from build123d import *
from OCP.BRepFilletAPI import BRepFilletAPI_MakeChamfer

# Parameters (mm, degrees)
SKETCH1_W               = 41
SKETCH1_H               = 34.5
SKETCH1_W_2             = 35
SKETCH1_H_2             = 28.5
BOSS_EXTRUDE1_DEPTH     = 5
SKETCH2_W               = 35
SKETCH2_H               = 28.5
BOSS_EXTRUDE2_DEPTH     = 1
SKETCH6_W               = 34.5
SKETCH6_H               = 5
CUT_EXTRUDE2_DEPTH      = 3
SKETCH7_W               = 1.6
SKETCH7_H               = 3
SKETCH7_H_2             = 3.078736203
BOSS_EXTRUDE3_DEPTH     = 4
CHAMFER1_SIZE           = 3
SKETCH14_W              = 3.502632447
SKETCH14_H              = 20.452559449
CUT_EXTRUDE6_DEPTH      = 10
BOSS_EXTRUDE5_DEPTH     = 4
BOSS_EXTRUDE7_DEPTH     = 1
SKETCH9_W               = 3.28281374
SKETCH9_H               = 22.420706044
CUT_EXTRUDE3_DEPTH      = 4
BOSS_EXTRUDE4_DEPTH     = 2
SKETCH12_W              = 3.28281374
SKETCH12_H              = 22.420706044
CUT_EXTRUDE4_DEPTH      = 0.003863752
BOSS_EXTRUDE8_DEPTH     = 2
BOSS_EXTRUDE9_DEPTH     = 2
CUT_EXTRUDE7_DEPTH      = 38.864903937
CUT_EXTRUDE7_DEPTH_BACK = 4
CHAMFER2_SIZE           = 3
CHAMFER2_SIZE_2         = 3.001586398
CHAMFER2_SIZE2          = 3
CHAMFER3_SIZE           = 2
BOSS_EXTRUDE10_DEPTH    = 7
CUT_EXTRUDE8_START      = -2
CUT_EXTRUDE8_DEPTH      = 7
CUT_EXTRUDE9_DEPTH      = 7
CUT_EXTRUDE11_START     = 1
CUT_EXTRUDE11_DEPTH     = 10
CUT_EXTRUDE12_DEPTH     = 10
SKETCH30_W              = 2.837179027
SKETCH30_H              = 7
CUT_EXTRUDE13_DEPTH     = 10
BOSS_EXTRUDE11_DEPTH    = 7
CUT_EXTRUDE14_DEPTH     = 7
SKETCH35_W              = 36.645868519
SKETCH35_H              = 38.499838471
CUT_EXTRUDE15_DEPTH     = 2
SKETCH37_W              = 2
SKETCH37_H              = 8.507497338
BOSS_EXTRUDE12_DEPTH    = 2
FILLET2_R               = 2


with BuildPart() as part:
    # Sketch1 → Boss-Extrude1 (new body)
    with BuildSketch(Plane(origin=(0, 0, 0), x_dir=(1, 0, 0), z_dir=(0, 1, 0))):
        with Locations((-14.14154724, 0.334775681)):
            Rectangle(SKETCH1_W, SKETCH1_H)
        with Locations((-14.14154724, 0.334775681)):
            Rectangle(SKETCH1_W_2, SKETCH1_H_2, mode=Mode.SUBTRACT)
    extrude(amount=BOSS_EXTRUDE1_DEPTH)

    # Sketch2 → Boss-Extrude2 (add)
    with BuildSketch(Plane(origin=(0, 0, 0), x_dir=(1, 0, 0), z_dir=(0, 1, 0))):
        with Locations((-14.14154724, 0.334775681)):
            Rectangle(SKETCH2_W, SKETCH2_H)
    extrude(amount=BOSS_EXTRUDE2_DEPTH)

    # Sketch6 → Cut-Extrude2 (cut)
    with BuildSketch(Plane.ZY.offset(34.64154724)):
        with Locations((-0.334775681, 2.5)):
            Rectangle(SKETCH6_W, SKETCH6_H)
    extrude(amount=-CUT_EXTRUDE2_DEPTH, mode=Mode.SUBTRACT)

    # Sketch7 → Boss-Extrude3 (add)
    with BuildSketch(Plane(origin=(0, 1, 0), x_dir=(1, 0, 0), z_dir=(0, 1, 0))):
        with Locations((-30.84154724, 13.084775681)):
            Rectangle(SKETCH7_W, SKETCH7_H)
        with Locations((-30.84154724, -12.375856218)):
            Rectangle(SKETCH7_W, SKETCH7_H_2)
    extrude(amount=BOSS_EXTRUDE3_DEPTH)

    # Chamfer1
    chamfer1_edges = [part.edges().sort_by_distance(p)[0] for p in [
        (-31.64154724, 2.5, -17.584775681),
        (-31.64154724, 2.5, 16.915224319),
        (6.35845276, 2.5, -17.584775681),
        (6.35845276, 2.5, 16.915224319),
    ]]
    chamfer(chamfer1_edges, length=CHAMFER1_SIZE)

    # Sketch14 → Cut-Extrude6 (cut)
    with BuildSketch(Plane(origin=(0, 1, 0), x_dir=(1, 0, 0), z_dir=(0, 1, 0))):
        with Locations((5.109768984, -7.134544415)):
            Rectangle(SKETCH14_W, SKETCH14_H)
    extrude(amount=CUT_EXTRUDE6_DEPTH, mode=Mode.SUBTRACT)

    # Sketch17 → Boss-Extrude5 (add)
    with BuildSketch(Plane(origin=(0, 1, 0), x_dir=(1, 0, 0), z_dir=(0, 1, 0))):
        Polygon((3.35845276, 3.09173531), (7.910000942, 0), (7.910000942, -13.915224319), (3.35845276, -13.915224319), (3.35845276, -16.915224319), (10.910000942, -16.915224319), (10.910000942, 3.419581668), (3.35845276, 8.549130391), align=None)
    extrude(amount=BOSS_EXTRUDE5_DEPTH)

    # Sketch19 → Boss-Extrude7 (add)
    with BuildSketch(Plane.XZ):
        Polygon((3.35845276, 16.915224319), (10.910000942, 16.915224319), (10.910000942, -3.419581668), (6.35845276, -6.511316978), (6.35845276, 13.915224319), align=None)
    extrude(amount=-BOSS_EXTRUDE7_DEPTH)

    # Sketch9 → Cut-Extrude3 (cut)
    with BuildSketch(Plane(origin=(0, 1, 0), x_dir=(1, 0, 0), z_dir=(0, 1, 0))):
        with Locations((-30.00014037, 0.374422659)):
            Rectangle(SKETCH9_W, SKETCH9_H)
    extrude(amount=-CUT_EXTRUDE3_DEPTH, mode=Mode.SUBTRACT)

    # Sketch11 → Boss-Extrude4 (add)
    with BuildSketch(Plane.XZ):
        Polygon((-26.665503706, 18.915224319), (-31.64154724, 13.915224319), (-31.64154724, -14.584775681), (-26.629189212, -19.584775681), (4.233785533, -19.584775681), (8.35845276, -15.460108453), (8.35845276, 14.743651444), (4.263960312, 18.915224319), align=None)
    extrude(amount=BOSS_EXTRUDE4_DEPTH)

    # Sketch12 → Cut-Extrude4 (cut)
    with BuildSketch(Plane(origin=(0, 0, 0), x_dir=(1, 0, 0), z_dir=(0, 1, 0))):
        with Locations((-30.00014037, 0.374422659)):
            Rectangle(SKETCH12_W, SKETCH12_H)
    extrude(amount=-CUT_EXTRUDE4_DEPTH, mode=Mode.SUBTRACT)

    # Sketch20 → Boss-Extrude8 (add)
    with BuildSketch(Plane.XZ):
        Polygon((6.227005221, 16.915224319), (10.910000942, 16.915224319), (10.910000942, -3.419581668), (8.35845276, -5.152774704), (8.35845276, 14.743651444), align=None)
    extrude(amount=BOSS_EXTRUDE8_DEPTH)

    # Sketch21 → Boss-Extrude9 (add)
    with BuildSketch(Plane(origin=(0, 0, 0), x_dir=(1, 0, 0), z_dir=(0, 1, 0))):
        Polygon((8.35845276, 7.570549944), (8.35845276, 5.152774704), (10.90766939, 3.421165424), (10.90766939, -16.912751148), (6.227005221, -16.915224319), (4.263960312, -18.915224319), (7.06681334, -18.91478086), (12.90766939, -18.911694666), (12.90766939, 4.480398389), align=None)
    extrude(amount=-BOSS_EXTRUDE9_DEPTH)

    # Sketch23 → Cut-Extrude7 (cut, two sides)
    with BuildSketch(Plane(origin=(0, 5, 0), x_dir=(1, 0, 0), z_dir=(0, 1, 0))) as cut_extrude7_sk:
        Polygon((7.910000942, 0), (7.910000942, 1.828776855), (3.35845276, 4.913740582), (3.35845276, 3.09173531), align=None)
    extrude(amount=CUT_EXTRUDE7_DEPTH, mode=Mode.SUBTRACT)
    extrude(cut_extrude7_sk.sketch, amount=-CUT_EXTRUDE7_DEPTH_BACK, mode=Mode.SUBTRACT)

    # Chamfer2: one chamfer whose edges measure the first distance from different faces: ONE call of the kernel's chamfer builder (chamfer() names one face for all edges)
    chamfer2_edges_1 = [part.edges().sort_by_distance(p)[0] for p in [
        (10.910000942, 2.5, 16.915224319),
    ]]
    chamfer2_edges_2 = [part.edges().sort_by_distance(p)[0] for p in [
        (12.90766939, -1, 18.911694666),
    ]]
    chamfer2_side_2 = [part.faces().sort_by_distance(p)[0] for p in [
        (9.987241365, -1, 18.913237763),
    ]]
    chamfer2 = BRepFilletAPI_MakeChamfer(part.part.solid().wrapped)
    for e in chamfer2_edges_1:
        chamfer2.Add(CHAMFER2_SIZE, e.wrapped)
    for e in chamfer2_edges_2:
        chamfer2.Add(CHAMFER2_SIZE_2, CHAMFER2_SIZE2, e.wrapped, chamfer2_side_2[0].wrapped)  # the first distance lies on this face
    add(Compound.cast(chamfer2.Shape()), mode=Mode.REPLACE)

    # Chamfer3
    chamfer3_edges = [part.edges().sort_by_distance(p)[0] for p in [
        (7.910000942, 3, 13.915224319),
    ]]
    chamfer(chamfer3_edges, length=CHAMFER3_SIZE)

    # Sketch25 → Boss-Extrude10 (add)
    with BuildSketch(Plane(origin=(0, 0, 0), x_dir=(1, 0, 0), z_dir=(0, 1, 0))):
        Polygon((-28.64154724, 17.584775681), (-26.629189212, 19.584775681), (4.233785533, 19.584775681), (8.35845276, 15.460108453), (8.35845276, 7.570549944), (12.90766939, 4.480398389), (12.90766939, -15.911694666), (9.906083411, -18.913280645), (-26.665503706, -18.915224319), (-28.64154724, -16.915224319), (7.910000942, -16.915224319), (10.910000942, -13.915224319), (10.910000942, 3.419581668), (6.35845276, 6.511316978), (6.35845276, 14.584775681), (3.35845276, 17.584775681), align=None)
    extrude(amount=BOSS_EXTRUDE10_DEPTH)

    # Sketch26 → Cut-Extrude8 (cut)
    with BuildSketch(Plane.XZ.offset(2).offset(CUT_EXTRUDE8_START)):
        Polygon((10.90766939, -3.421165424), (10.90766939, 15.083267541), (9.077218609, 16.913718322), (7.066126742, 16.914780944), (4.263802095, 16.915224319), (-25.834261771, 16.915224319), (-29.64154724, 13.089609206), (-29.64154724, -13.754902141), (-25.802207763, -17.584775681), (3.405358408, -17.584775681), (6.35845276, -14.631681329), (6.35845276, -6.511316978), align=None)
    extrude(amount=-CUT_EXTRUDE8_DEPTH, mode=Mode.SUBTRACT)

    # Sketch27 → Cut-Extrude9 (cut)
    with BuildSketch(Plane(origin=(0, 0, 0), x_dir=(1, 0, 0), z_dir=(0, 1, 0))):
        Polygon((-25.802207763, 17.584775681), (-28.64154724, 17.584775681), (-31.64154724, 14.584775681), (-31.64154724, 11.584775681), (-29.64154724, 11.584775681), (-29.64154724, 13.754902141), align=None)
        Polygon((-29.64154724, -10.835930363), (-29.64154724, -13.089609206), (-25.834261771, -16.915224319), (-28.64154724, -16.915224319), (-31.64154724, -13.915224319), (-31.64154724, -10.835930363), align=None)
    extrude(amount=CUT_EXTRUDE9_DEPTH, mode=Mode.SUBTRACT)

    # Sketch28 → Cut-Extrude11 (cut)
    with BuildSketch(Plane(origin=(0, -0.003863752, 0), x_dir=(1, 0, 0), z_dir=(0, 1, 0)).offset(CUT_EXTRUDE11_START)):
        Polygon((-31.64154724, -13.915224319), (-26.665503706, -18.915224319), (9.906083411, -18.913280645), (12.90766939, -15.911694666), (12.90766939, 4.480398389), (8.35845276, 7.570549944), (8.35845276, 15.460108453), (4.233785533, 19.584775681), (-26.629189212, 19.584775681), (-31.64154724, 14.584775681), align=None)
    extrude(amount=CUT_EXTRUDE11_DEPTH, mode=Mode.SUBTRACT)

    # Sketch29 → Cut-Extrude12 (cut)
    with BuildSketch(Plane(origin=(0, -0.003863752, 0), x_dir=(1, 0, 0), z_dir=(0, 1, 0))):
        Polygon((-31.64154724, 14.584775681), (-26.629189212, 19.584775681), (4.233785533, 19.584775681), (8.35845276, 15.460108453), (8.35845276, 7.570549944), (12.90766939, 4.480398389), (12.90766939, -15.911694666), (9.906083411, -18.913280645), (-26.665503706, -18.915224319), (-31.64154724, -13.915224319), align=None)
    extrude(amount=CUT_EXTRUDE12_DEPTH, mode=Mode.SUBTRACT)


with BuildPart() as cut_extrude12_piece_1:
    # of the separate pieces the step leaves, piece 1, a body of its own (cut_extrude12_pieces)
    add(part.part.solids().sort_by_distance((-31.64154724, -0.003863752, -14.584775681))[0])

    # Sketch31 → Boss-Extrude11 (add)
    with BuildSketch(Plane.XZ.offset(2)):
        Polygon((6.35845276, -6.511316978), (10.90766939, -3.421165424), (10.90766939, 15.083267541), (9.077218609, 16.913718322), (7.066126742, 16.914780944), (4.263802095, 16.915224319), (-25.834261771, 16.915224319), (-29.64154724, 13.089609206), (-31.64154724, 13.915224319), (-26.665503706, 18.915224319), (9.906083411, 18.913280645), (12.90766939, 15.911694666), (12.90766939, -4.480398389), (8.35845276, -7.570549944), (8.35845276, -15.460108453), (4.233785533, -19.584775681), (-26.629189212, -19.584775681), (-31.64154724, -14.584775681), (-29.64154724, -13.754902141), (-25.802207763, -17.584775681), (3.405358408, -17.584775681), (6.35845276, -14.631681329), align=None)
    extrude(amount=BOSS_EXTRUDE11_DEPTH)

    # Sketch32 → Cut-Extrude14 (cut)
    with BuildSketch(Plane.XZ.offset(2)):
        Polygon((-25.834261771, 16.915224319), (-25.802207763, -17.584775681), (-29.64154724, -13.754902141), (-31.64154724, -14.584775681), (-31.64154724, 13.915224319), (-29.64154724, 13.089609206), align=None)
        Polygon((-29.64154724, 13.089609206), (-25.834261771, 16.915224319), (-36.844784184, 16.915224319), (-37.593826415, -17.584775681), (-25.802207763, -17.584775681), (-29.64154724, -13.754902141), (-31.64154724, -14.584775681), (-31.64154724, 13.915224319), align=None)
    extrude(amount=CUT_EXTRUDE14_DEPTH, mode=Mode.SUBTRACT)

    # Sketch35 → Cut-Extrude15 (cut)
    with BuildSketch(Plane.XZ.offset(9)):
        with Locations((-5.303289834, -0.334856445)):
            Rectangle(SKETCH35_W, SKETCH35_H)
    extrude(amount=-CUT_EXTRUDE15_DEPTH, mode=Mode.SUBTRACT)

    # Sketch37 → Boss-Extrude12 (add)
    with BuildSketch(Plane.XZ.offset(7)):
        with Locations((11.90766939, 5.829727419)):
            Rectangle(SKETCH37_W, SKETCH37_H)
    extrude(amount=BOSS_EXTRUDE12_DEPTH)

    # Fillet2
    fillet2_edges = [cut_extrude12_piece_1.edges().sort_by_distance(p)[0] for p in [
        (12.90766939, -3.501931876, -4.480398389),
        (8.35845276, -3.501931876, -7.570549944),
        (4.233785533, -3.501931876, -19.584775681),
        (8.35845276, -3.501931876, -15.460108453),
        (12.90766939, -3.501931876, 15.911694666),
    ]]
    fillet(fillet2_edges, radius=FILLET2_R)


with BuildPart() as cut_extrude12_piece_2:
    # of the separate pieces the step leaves, piece 2, a body of its own (cut_extrude12_pieces)
    add(part.part.solids().sort_by_distance((-28.634132423, 0, -17.584775681))[0])

    # Sketch30 → Cut-Extrude13 (cut)
    with BuildSketch(Plane(origin=(-23.02477977, 0, -23.167050199), x_dir=(-0.7092812996014342, 0, 0.7049255549600261), z_dir=(-0.7049255549600261, 0, -0.7092812996014342))):
        with Locations((6.500366579, 3.5)):
            Rectangle(SKETCH30_W, SKETCH30_H)
    extrude(amount=-CUT_EXTRUDE13_DEPTH, mode=Mode.SUBTRACT)


solid = cut_extrude12_piece_1.part
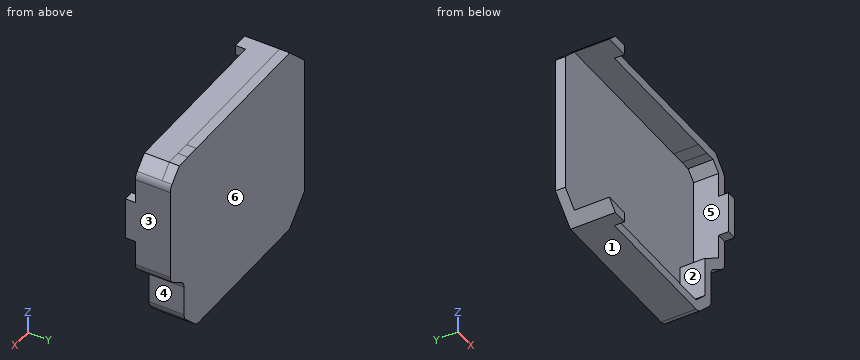
Input: part model. Units: mm. Frame: model coordinates. Face numbers are marked on the shaded views. A direction names the side the tool comes from. Give positions to 0.01 mm unless a question says otherwise; leave off trailing zeros. Loops run counter-clockwise (first coordinate to the right, second up) from the corner with the lowest first, then second, coordinate; pieces in that order, holes last. Notation, with made-up numbers: (39.25, 10.5) - (51.25, 10.5) arc R33 ccw to (51.25, 47.5) - close; hole circle Ø4 at (-5.5, 85). An arc over 180 degrees is marked (long way). Use CSV: the item, a comma, the result in double quotes. Start each with the question number.
Item 1: Line query: line 1 (Z direction, x = -5, y = -4.5); line 2 (X direction, y = -6, z = 0.5); line 3 (Y direction, x = -20.5, z = -9.5). Output: solid intervals per line, ascending.
Item 2: Section D-D on y = -4. Return loops of the section in (x, z).
Item 3: Section B-B on z = 2.5. Return loops of the section in (x, y).
Item 4: Mould query, pull axis Z, two halves, no side actions, for the marked faces 1, 2 and 3. Classes: pulls with the +Z half, pulls with the -Z half, needs draft (parallel to the pull), parting line crosses it, or undercut.
Item 5: Section A-A on y = -1.25. Return loops of the section in (x, z).
Item 6: Contact query for flat-ended pins moving along their axis: P1, Ø1.5, axis at x = -15, z = 2, coming from the +Y side; P2, Ø10.5, axis at x = -20, z = -1, coming from the -Y side; P3, Ø12, axis at x = 3.5, z = -15, coming from the -Y side. Output: stop coordinate, or through.
Item 7: Reachability of the marked faces 4, 5 and 6 from +Z, -Z, +X, -X, +Y, -Y: full face, straight path, thin tool, end or side. Return the list, or none.
Ans:
1,line 1,"z = -19.58 to -17.58, 16.92 to 18.91"
1,line 2,"x = 10.91 to 12.91"
1,line 3,"y = -2 to 0"
2,outline,"(-28.66, 16.92) - (4.26, 16.92) - (7.07, 16.91) - (9.08, 16.91) - (10.91, 15.08) - (10.91, -3.42) - (6.36, -6.51) - (6.36, -14.63) - (3.41, -17.58) - (-28.63, -17.58) - (-26.63, -19.58) - (3.41, -19.58) arc R2 ccw to (4.82, -19) - (7.77, -16.05) arc R2 ccw to (8.36, -14.63) - (8.36, -8.63) arc R2 cw to (9.23, -6.98) - (12.03, -5.08) arc R2 ccw to (12.91, -3.42) - (12.91, 15.08) arc R2 ccw to (12.32, 16.5) - (9.91, 18.91) - (-26.67, 18.92) - close"
3,outline,"(-31.64, -2) - (10.91, -2) - (10.91, -9) - (12.91, -9) - (12.91, 0) - (-31.64, 0) - close"
4,face 1,"pulls with the -Z half"
4,face 2,"undercut"
4,face 3,"needs draft"
5,outline,"(-31.64, -14.58) - (-26.63, -19.58) - (3.41, -19.58) arc R2 ccw to (4.82, -19) - (7.77, -16.05) arc R2 ccw to (8.36, -14.63) - (8.36, -8.63) arc R2 cw to (9.23, -6.98) - (12.03, -5.08) arc R2 ccw to (12.91, -3.42) - (12.91, 15.08) arc R2 ccw to (12.32, 16.5) - (9.91, 18.91) - (7.07, 18.91) - (4.26, 18.92) - (-26.67, 18.92) - (-31.64, 13.92) - close"
6,P1,"stops at y = 0"
6,P2,"stops at y = -2"
6,P3,"stops at y = -7"
7,face 4,"-Z, +X, +Y, -Y"
7,face 5,"-X, -Y"
7,face 6,"+Z, -Z, +X, -X, +Y"
